Work out the finished part from the listing and answer in its coordinate system (mm). A direction names the side the tool comes from. Coordinates: 2 decimals unless noted, no trailing zeros. Order: outer loops, then holes, each group sorted by start corner. A loop starts at its lowest first (then second) coordinate and runs counter-clockwise, first axis right, second up. Notation, with made-up numbers: M 68.5,38.5 L 92.5,38.5 A11 cw 92.5,59.5 Z; hole C -39.5,-21 d8. An arc over 180 degrees is marked long. Use a Markdown table: item, result. Add a question column.
Autodesk Inventor part; units mm, degrees
ref_plane "YZ Plane" through (0, 0, 0) normal (1, 0, 0) x (0, 1, 0)
ref_plane "XZ Plane" through (0, 0, 0) normal (0, 1, 0) x (-1, 0, 0)
ref_plane "XY Plane" through (0, 0, 0) normal (0, 0, 1) x (1, 0, 0)
sketch "Skizze1" plane through (0, 0, 0) normal (0, 0, 1) x (1, 0, 0)
  line L0 (-100, 0) -> (100, 0)
  line L1 (100, 0) -> (100, 140)
  line L2 (100, 140) -> (-100, 140)
  line L3 (-100, 140) -> (-100, 0)
  point P0 (0, 0)
  dimension "d0" = 200
  dimension "d1" = 140
extrude "Extrusion1" add sketch "Skizze1" along normal blind 200
sketch "Skizze2" plane through (-100, 140, 0) normal (0, 1, 0) x (1, 0, 0)
  circle A0 centre (100, -250) radius 100
  point P0 (100, 0)
  dimension "d4" = 200
extrude "Extrusion2" cut sketch "Skizze2" against normal blind 140
sketch "Skizze3" plane through (0, 0, 0) normal (0, 0, -1) x (-1, 0, 0)
  point P0 (0, 0)
sketch "Skizze4" plane through (0, 0, 0) normal (0, 0, -1) x (-1, 0, 0)
  line L0 (15, 68) -> (-15, 68)
  line L1 (-15, 68) -> (-15, 60)
  line L2 (-15, 60) -> (15, 60)
  line L3 (15, 60) -> (15, 68)
  line L4 (-15, 76) -> (15, 76)
  line L5 (15, 76) -> (15, 84)
  line L6 (15, 84) -> (-15, 84)
  line L7 (-15, 84) -> (-15, 76)
  line L8 (-15, 92) -> (15, 92)
  line L9 (15, 92) -> (15, 100)
  line L10 (15, 100) -> (-15, 100)
  line L11 (-15, 100) -> (-15, 92)
  point P0 (0, 0)
  dimension "d7" = 30
  dimension "d8" = 8
  dimension "d9" = 30
  dimension "d10" = 8
  dimension "d11" = 8
extrude "Extrusion3" add sketch "Skizze4" along normal blind 60
sketch "Skizze5" plane through (-15, 100, 0) normal (0, 1, 0) x (1, 0, 0)
  circle A0 centre (15, 30) radius 7
  line L0 (0, 60) -> (30, 60)
  arc A1 (30, 60) -> (0, 60) centre (15, 60) ccw
  point P0 (15, 0)
  dimension "d14" = 14
  dimension "d15" = 15
extrude "Extrusion4" cut sketch "Skizze5" against normal blind 40 contours A0
sketch "Skizze6" plane through (0, 0, 0) normal (0, 0, -1) x (-1, 0, 0)
  line L0 (-100, 0) -> (-100, 140)
  line L1 (100, 140) -> (100, 0)
  line L2 (-100, 140) -> (100, 140)
  line L3 (100, 140) -> (100, 125)
  line L4 (100, 125) -> (-100, 125)
  line L5 (-100, 125) -> (-100, 140)
  point P0 (0, 0)
  dimension "d18" = 15
extrude "Extrusion5" add sketch "Skizze6" along normal blind 140
properties part number "Ausschub_Magazin"
(1) A cutting plane is placed at D-D on x = 27. Write down the section's boundary in (y, z).
(2) Which of the six approach directions +Z, -Z, +X, -X, +Y, -Y give full straight-line access (tool end or side, diameter ignored) to faces 1 (the flat face through (15, 96, -30)), 2 (the flat face through (-15, 64, -30)), 3 (the flat face through (0, 96, -60)), 4 (the flat face through (100, 69, 108)), 5 (the flat face through (4, 92, -23))?
(3) A cutting plane is placed at B-B on x = -1. Count the separate pieces of the cut face and the enclosed holes in it, plus the area to 3 significant figures.
(4) A cutting plane is placed at A-A on z = -30. Write down the section's boundary in (x, y), plus the area to 3 significant figures.
(5) Given P1, Ø6.5, axis at y = 62, z = -17, coming from the -X side; P2, Ø6.5, axis at y = 78, z = -38.5, coming from the +X side; P3, Ø8, axis at x = -41.5, y = 29.5, coming from the -Z side; P4, Ø3, axis at x = 13.5, z = 130, coming from the -Y side, each flat-ended and moving along its own axis, determine where each tip first touches the part or whether it passes through.
(6) The mould has two halves that part along X. Classify faces 6 (the flat face through (-15, 96, -30)), 7 (the flat face through (93, 71, 200)), 8 (the cylindrical face through (-1.517, 64.056, -23.166)), 9 (the cylindrical face through (-1.517, 96.056, -23.166)): pulls with the +X half, pulls with the -X half, needs draft (parallel to the pull), parting line crosses it, or undercut.
(7) A cutting plane is placed at C-C on y = 50. Write down the section's boundary in (x, z).
(8) Straight lines are drawn through the part: line 1 (Z direction, x = 0, y = 82); line 2 (X direction, y = 97.5, z = -30); line 3 (Y direction, x = 72, z = -76.5). For each, find the intervals that lie inside material, in ascending order.
From the geometry:
| question | item | result |
|---|---|---|
| 1 | outline | M 0,0 L 125,0 L 125,-140 L 140,-140 L 140,153.71 L 0,153.71 Z |
| 2 | face 1 | -Z, +X, -Y |
| 2 | face 2 | -Z, -X, -Y |
| 2 | face 3 | -Z, +X, -X, -Y |
| 2 | face 4 | +Z, -Z, +X, +Y, -Y |
| 2 | face 5 | -Z, +X, -X |
| 3 | separate pieces | 4 |
| 3 | enclosed holes | 0 |
| 3 | area | 24,200 mm2 |
| 4 | outline | M -100,125 L 100,125 L 100,140 L -100,140 Z; M -15,60 L -7,60 L -7,68 L -15,68 Z; M -15,76 L -7,76 L -7,84 L -15,84 Z; M -15,92 L -7,92 L -7,100 L -15,100 Z; M 7,60 L 15,60 L 15,68 L 7,68 Z; M 7,76 L 15,76 L 15,84 L 7,84 Z; M 7,92 L 15,92 L 15,100 L 7,100 Z |
| 4 | area | 3,380 mm2 |
| 5 | P1 | stops at x = -15 |
| 5 | P2 | stops at x = 15 |
| 5 | P3 | stops at z = 0 |
| 5 | P4 | stops at y = 0 |
| 6 | face 6 | pulls with the -X half |
| 6 | face 7 | needs draft |
| 6 | face 8 | undercut |
| 6 | face 9 | undercut |
| 7 | outline | M -100,0 L 100,0 L 100,200 L 86.6,200 A100 cw -86.6,200 L -100,200 Z |
| 8 | line 1 | z = -60 to -37, -23 to 150 |
| 8 | line 2 | x = -15 to -7, 7 to 15 |
| 8 | line 3 | y = 125 to 140 |
